Study the drawing (mm; zero at the part's minimum x, y, z) and answer. Give positions to 0.01 mm unless a question says otherwise; leave off trailing zeros. Loops run counter-clockwise (first coordinate to the right, second up) from the corner with the lowest first, then second, coordinate; pieces in that order, holes last. Notation, with made-up numbers: M -8.5,-17 L 33.5,-17 A21 cw 33.5,-6 Z; hole C 56.5,65.25 d8. An arc over 180 degrees is marked long. Use one line per item in the form item = value. Start each with the question number.
1. Each of these flat-tipped pins is pushed along its axis until it touches: pin 1 Ø10 at (y, z) = (87, 341) entering from -X; pin 2 Ø12 at (y, z) = (100.5, 352) entering from +X; pin 3 Ø3 at (x, y) = (152.5, 104) entering from -Z. Where does it stop, or does it pass through?
2. Straight lines are drawn through the part: line 1 (Z direction, x = 100, y = 59); line 2 (Z direction, x = 83, y = 126); line 3 (Z direction, x = 24, y = 103.5). For each, find the intervals that lie inside material, in ascending order. Write a range as from..to.
3. The part is cut by section A-A (x = 100). Write down the section's boundary in (y, z), and give its area (3 significant figures).
4. The part is cut by section D-D (z = 32). Write down the section's boundary in (x, y), and give its area (3 significant figures).
5. The part is cut by section B-B (z = 200). Write down the section's boundary in (x, y), and give its area (3 significant figures).
6. The mould has two halves that part along X. Classify the marked faces 1, 2 and 3: released by +X, released by -X, zero draft, split by the parting line, or undercut.
7. The part is cut by section C-C (y = 16). Write down the section's boundary in (x, z).
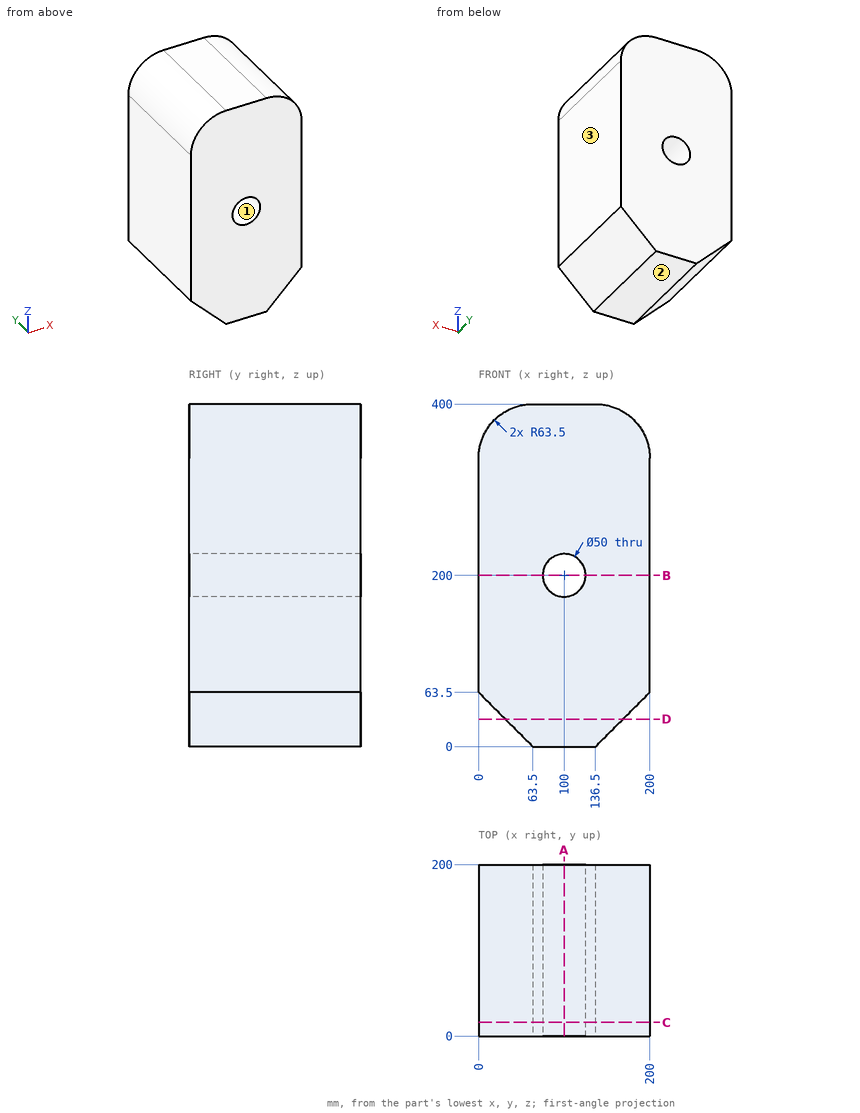
Derived:
q1.pin_1 = 0
q1.pin_2 = 199.29
q1.pin_3 = 14.5
q2.line_1 = 0..175, 225..400
q2.line_2 = 0..181.67, 218.33..400
q2.line_3 = 39.5..386.22
q3.outline = M 0,0 L 200,0 L 200,175 L 0,175 Z; M 0,225 L 200,225 L 200,400 L 0,400 Z
q3.area = 70,000 mm2
q4.outline = M 31.5,0 L 168.5,0 L 168.5,200 L 31.5,200 Z
q4.area = 27,400 mm2
q5.outline = M 0,0 L 75,0 L 75,200 L 0,200 Z; M 125,0 L 200,0 L 200,200 L 125,200 Z
q5.area = 30,000 mm2
q6.face_1 = undercut
q6.face_2 = zero draft
q6.face_3 = released by +X
q7.outline = M 0,63.5 L 63.5,0 L 136.5,0 L 200,63.5 L 200,336.5 A63.5 ccw 136.5,400 L 63.5,400 A63.5 ccw 0,336.5 Z; hole C 100,200 d50
